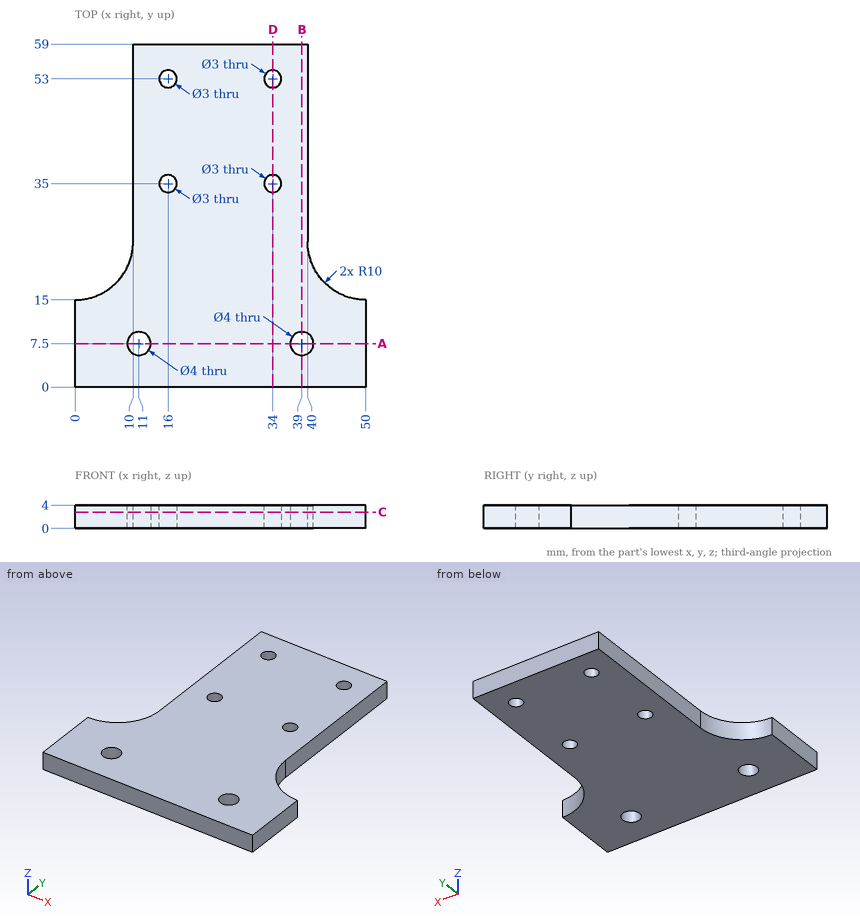
The drawing under review shows one solid part. Ordinate dimensions are in mm from its lowest x, y, z. Give positions to 0.01 mm unless a question says otherwise; leave off trailing zeros. Write each loop counter-clockwise with the first axis right and the second up, starting at its lowest first coordinate (ties: lowest second). Pieces come first, ordered by that corner, then holes.
1. Add section A-A, the plane y = 7.5. Write out the cut boundary in (x, z), plus the area to 3 significant figures.
2. Add section B-B, the plane x = 39. Write out the cut boundary in (y, z).
3. Add section D-D, the plane x = 34. Write out the cut boundary in (y, z).
4. For P1, Ø1, axis at y = 51, z = 0.5, coming from the +X side, flat-tipped, find the tip position at first contact; note if it passes through.
5. Wall thickness on L1, parallel to Y at x = 34, z = 3.15; L2, parallel to Y at x = 11, z = 3.05; L3, parallel to X at y = 39.5, z = 2.9: over which ranges is each line inside the solid? List them lowest first.
6. Add section C-C, the plane z = 2.8. Count the separate pieces of the cut face and the enclosed holes in it, plus the area to 3 significant figures.
Worked answers:
1. outline: (0, 0) - (9, 0) - (9, 4) - (0, 4) - close; (13, 0) - (37, 0) - (37, 4) - (13, 4) - close; (41, 0) - (50, 0) - (50, 4) - (41, 4) - close
1. area: 168 mm2
2. outline: (0, 0) - (5.5, 0) - (5.5, 4) - (0, 4) - close; (9.5, 0) - (59, 0) - (59, 4) - (9.5, 4) - close
3. outline: (0, 0) - (33.5, 0) - (33.5, 4) - (0, 4) - close; (36.5, 0) - (51.5, 0) - (51.5, 4) - (36.5, 4) - close; (54.5, 0) - (59, 0) - (59, 4) - (54.5, 4) - close
4. P1: stops at x = 40
5. L1: y = 0 to 33.5, 36.5 to 51.5, 54.5 to 59
5. L2: y = 0 to 5.5, 9.5 to 59
5. L3: x = 10 to 40
6. separate pieces: 1
6. enclosed holes: 6
6. area: 2,060 mm2
